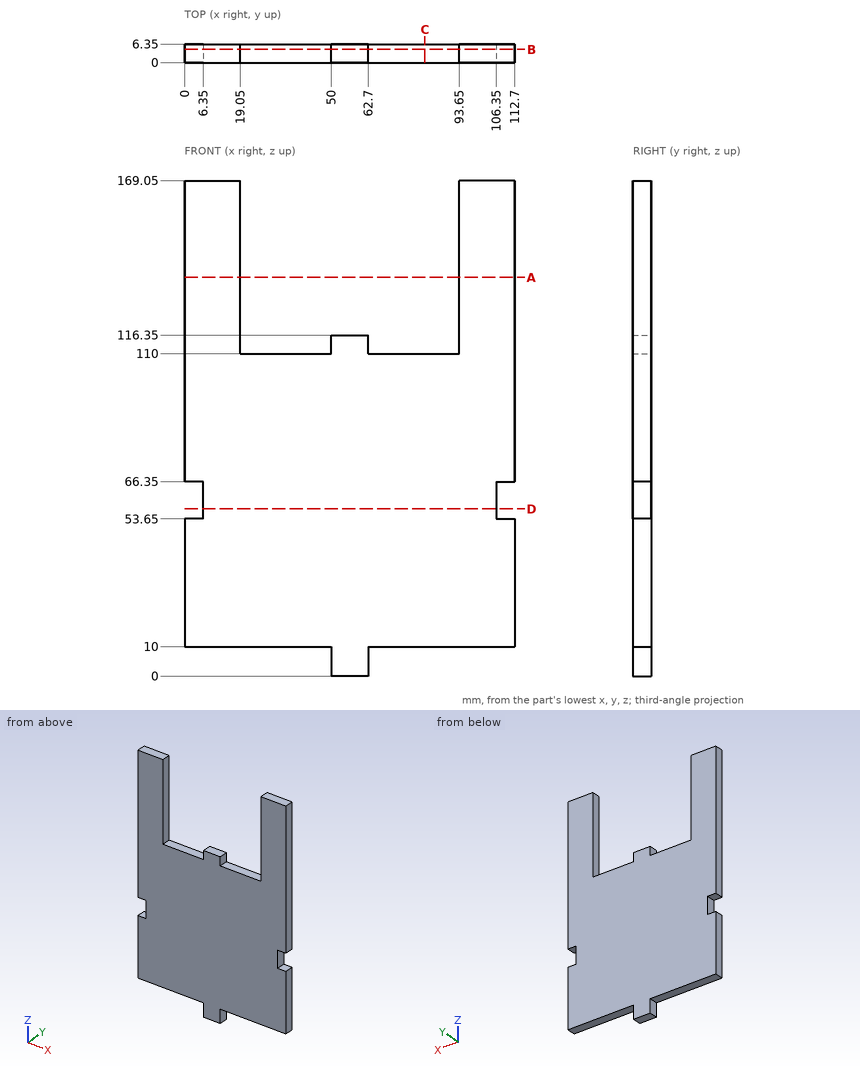
The figure shows three views and two pictorial views of one solid part (mm, origin at its lowest corner). Answer the questions. Give positions to 0.01 mm unless a question says otherwise; leave off trailing zeros. Write each loop counter-clockwise with the first axis right and the second up, starting at its lowest first coordinate (ties: lowest second). Pieces come first, ordered by that corner, then holes. Notation, with made-up numbers: M 44,-15 L 81,-15 A18 ccw 81,18 Z; hole C -34,7 d6. An arc over 180 degrees is marked long. One line per item, written item: value. Start each with the question number.
(1) Find section D-D (z = 57). Determine the outline of the cut face in (x, y).
(2) Find section A-A (z = 136). Determine the outline of the cut face in (x, y).
(3) Find the intervals of material crossed by line 1 (X direction, y = 4, z = 114); line 2 (X direction, y = 1.5, z = 125.5); line 3 (Z direction, x = 27, y = 5), in increasing order.
(4) Find section B-B (y = 4.5). Determine the outline of the cut face in (x, z), plus the area to 3 significant figures.
(5) Flat-ended cylindrical pins translate along their axes: pin 1 Ø3 at (x, y) = (77.5, 4.5) entering from -Z; pin 2 Ø3 at (x, y) = (86, 2.5) entering from +Z; pin 3 Ø3 at (y, z) = (2, 4.5) entering from -X. Find the tip coordinate at first contact, or state that the pin passes through.
(6) Find section C-C (x = 82). Determine the outline of the cut face in (y, z), plus the area to 3 significant figures.
Results below:
1. outline: M 6.35,0 L 106.35,0 L 106.35,6.35 L 6.35,6.35 Z
2. outline: M 0,0 L 19.05,0 L 19.05,6.35 L 0,6.35 Z; M 93.65,0 L 112.7,0 L 112.7,6.35 L 93.65,6.35 Z
3. line 1: x = 0 to 19.05, 50 to 62.7, 93.65 to 112.7
3. line 2: x = 0 to 19.05, 93.65 to 112.7
3. line 3: z = 10 to 110
4. outline: M 0,10 L 50,10 L 50,0 L 62.7,0 L 62.7,10 L 112.7,10 L 112.7,53.65 L 106.35,53.65 L 106.35,66.35 L 112.7,66.35 L 112.7,169.05 L 93.65,169.05 L 93.65,110 L 62.7,110 L 62.7,116.35 L 50,116.35 L 50,110 L 19.05,110 L 19.05,169.05 L 0,169.05 L 0,66.35 L 6.35,66.35 L 6.35,53.65 L 0,53.65 Z
4. area: 13,600 mm^2
5. pin 1: stops at z = 10
5. pin 2: stops at z = 110
5. pin 3: stops at x = 50
6. outline: M 0,10 L 6.35,10 L 6.35,110 L 0,110 Z
6. area: 635 mm^2
